Source: CAD feature listing. Evaluate the final solid. Frame: model axes, mm. A direction names the side the tool comes from. Coordinates: 2 decimals unless noted, no trailing zeros. Order: outer loops, then holes, each group sorted by start corner. A loop starts at its lowest first (then second) coordinate and runs counter-clockwise, first axis right, second up. Notation, with made-up numbers: (-39.75, 41) - (-1.75, 41) arc R30 ccw to (-1.75, 63) - close; hole circle Ø10 at (87, 77.5). An arc over 180 degrees is marked (long way). One line per question, with ' | ' between items. Start each with the question number.
(1) Section A-A (z = 0). Return the cut outline in (x, y).
(2) Section D-D (z = -46). Return the cut outline in (x, y).
(3) Access query for faces 1 (the flat face through (-251, 6, -88.9)), 2 (the flat face through (-251, 265.545, -92)), 3 (the flat face through (-251, 132.773, 92)). Directions: +Z, -Z, +X, -X, +Y, -Y. A direction counts if a zero-diameter tool reaches every point of the face in a straight line with its end or side. Return the directions, or none.
(4) Contact query for flat-ended pins moving along their axis: P1, Ø1.5, axis at x = -249, y = 214.5, coming from the -Z side; P2, Ø1.9, axis at x = -251, z = -92, coming from the -Y side; P3, Ø3, axis at x = -251.5, z = -92.5, coming from the +Y side; P4, Ø5, axis at y = 92.583, z = -37.211, coming from the -X side. Output: stop coordinate, or through.
(5) Section B-B (y = 59.5). Return the cut outline in (x, z), then the cut area to 3 significant figures.
(6) Draft query along Y for faces 4 (the flat face through (-251, 225.136, 92)), 5 (the flat face through (-251, 292.1, 92)), 6 (the flat face through (-251, 0, -86)), 7 (the flat face through (-251, 20, -95.25)). Return one class per face: +Y half, -Y half, draft (parallel to the pull), parting line (faces both ways), or undercut.
(7) Section C-C (y = 162.5). Return the cut outline in (x, z), then the cut area to 3 significant figures.
(8) Line query: line 1 along Y through (x, z) = (-248.75, 47.5); line 2 along Y through (x, z) = (-251, 17); line 3 along Y through (x, z) = (-250.25, 22.5). Output: solid intervals per line, ascending.
from build123d import *

# Parameters (mm, degrees)
SKETCH1_W           = 508
SKETCH1_H           = 190.5
BOSS_EXTRUDE1_DEPTH = 6.35
SKETCH2_W           = 508
SKETCH2_H           = 190.5
SKETCH2_W_2         = 495.3
SKETCH2_H_2         = 177.8
BOSS_EXTRUDE2_DEPTH = 298.45
SKETCH3_W           = 6.35
SKETCH3_H           = 16.933333333
SKETCH3_H_2         = 16.933333334
CUT_EXTRUDE1_DEPTH  = 12.7
SKETCH4_W           = 6.35
SKETCH4_H           = 15.875
CUT_EXTRUDE2_DEPTH  = 6.35
SKETCH6_W           = 514.801062296
SKETCH6_H           = 254.881465808
CUT_EXTRUDE5_DEPTH  = 305.8
SKETCH5_W           = 6.35
SKETCH5_H           = 16.933333333
SKETCH5_H_2         = 16.933333334
CUT_EXTRUDE6_DEPTH  = 6.35
SKETCH7_W           = 6.35
SKETCH7_H           = 12.7
CUT_EXTRUDE7_DEPTH  = 7.35
SKETCH8_R           = 26.9875
SKETCH8_R_2         = 3.175
CUT_EXTRUDE8_DEPTH  = 7.35


with BuildPart() as part:
    # Sketch1 → Boss-Extrude1 (new body)
    with BuildSketch(Plane(origin=(0, 0, 0), x_dir=(1, 0, 0), z_dir=(0, 1, 0))):
        Rectangle(SKETCH1_W, SKETCH1_H)
    extrude(amount=BOSS_EXTRUDE1_DEPTH)

    # Sketch2 → Boss-Extrude2 (add)
    with BuildSketch(Plane(origin=(0, 6.35, 0), x_dir=(1, 0, 0), z_dir=(0, 1, 0))):
        Rectangle(SKETCH2_W, SKETCH2_H)
        Rectangle(SKETCH2_W_2, SKETCH2_H_2, mode=Mode.SUBTRACT)
    extrude(amount=BOSS_EXTRUDE2_DEPTH)

    # Sketch3 → Cut-Extrude1 (cut)
    with BuildSketch(Plane.XY.offset(95.25)):
        with BuildLine():
            Line((-3.302, 283.21), (-3.302, 6.35))
            Line((-3.302, 6.35), (3.302, 6.35))
            Line((3.302, 6.35), (3.302, 292.354))
            Line((3.302, 292.354), (-16.256, 292.354))
            Line((-16.256, 292.354), (-16.256, 285.75))
            Line((-16.256, 285.75), (-5.842, 285.75))
            ThreePointArc((-5.842, 285.75), (-4.045948776, 285.006051224), (-3.302, 283.21))
        make_face()
        with Locations((12.827, 80.433333334)):
            Rectangle(SKETCH3_W, SKETCH3_H)
        with Locations((12.827, 50.8)):
            Rectangle(SKETCH3_W, SKETCH3_H_2)
        with Locations((12.827, 21.166666667)):
            Rectangle(SKETCH3_W, SKETCH3_H)
    extrude(amount=-CUT_EXTRUDE1_DEPTH, mode=Mode.SUBTRACT)

    # Sketch4 → Cut-Extrude2 (cut)
    with BuildSketch(Plane.XY.offset(-88.9)):
        with Locations((-19.431, 284.1625)):
            Rectangle(SKETCH4_W, SKETCH4_H)
        with Locations((-19.431, 255.5875)):
            Rectangle(SKETCH4_W, SKETCH4_H)
        with Locations((-19.431, 227.0125)):
            Rectangle(SKETCH4_W, SKETCH4_H)
        with Locations((-19.431, 198.4375)):
            Rectangle(SKETCH4_W, SKETCH4_H)
        with Locations((-19.431, 169.8625)):
            Rectangle(SKETCH4_W, SKETCH4_H)
        with Locations((-19.431, 141.2875)):
            Rectangle(SKETCH4_W, SKETCH4_H)
        with Locations((-19.431, 112.7125)):
            Rectangle(SKETCH4_W, SKETCH4_H)
        with Locations((-19.431, 84.1375)):
            Rectangle(SKETCH4_W, SKETCH4_H)
        with Locations((-19.431, 55.5625)):
            Rectangle(SKETCH4_W, SKETCH4_H)
        with Locations((-19.431, 26.9875)):
            Rectangle(SKETCH4_W, SKETCH4_H)
    cut_extrude2 = extrude(amount=-CUT_EXTRUDE2_DEPTH, mode=Mode.SUBTRACT)

    # Mirror1: Cut-Extrude2 across plane
    add(cut_extrude2.mirror(Plane.ZY.offset(6.477)), mode=Mode.SUBTRACT)

    # Sketch6 → Cut-Extrude5 (cut, through all)
    with BuildSketch(Plane(origin=(0, 0, 0), x_dir=(1, 0, 0), z_dir=(0, 1, 0))):
        with Locations((9.750531148, -10.000845247)):
            Rectangle(SKETCH6_W, SKETCH6_H)
    extrude(amount=CUT_EXTRUDE5_DEPTH, mode=Mode.SUBTRACT)

    # Sketch5 → Cut-Extrude6 (cut)
    with BuildSketch(Plane(origin=(0, 0, 0), x_dir=(-1, 0, 0), z_dir=(0, -1, 0))):
        with Locations((250.825, -74.083333334)):
            Rectangle(SKETCH5_W, SKETCH5_H)
        with Locations((250.825, -44.45)):
            Rectangle(SKETCH5_W, SKETCH5_H_2)
        with Locations((250.825, -14.816666667)):
            Rectangle(SKETCH5_W, SKETCH5_H)
        with Locations((250.825, 14.816666667)):
            Rectangle(SKETCH5_W, SKETCH5_H)
        with Locations((250.825, 44.45)):
            Rectangle(SKETCH5_W, SKETCH5_H_2)
        with Locations((250.825, 74.083333334)):
            Rectangle(SKETCH5_W, SKETCH5_H)
    extrude(amount=-CUT_EXTRUDE6_DEPTH, mode=Mode.SUBTRACT)

    # Sketch7 → Cut-Extrude7 (cut, through all)
    with BuildSketch(Plane.ZY.offset(254)):
        with Locations((-92.075, 32.904545455)):
            Rectangle(SKETCH7_W, SKETCH7_H)
        with Locations((-92.075, 6.35)):
            Rectangle(SKETCH7_W, SKETCH7_H)
        with Locations((-92.075, 59.459090909)):
            Rectangle(SKETCH7_W, SKETCH7_H)
        with Locations((-92.075, 86.013636364)):
            Rectangle(SKETCH7_W, SKETCH7_H)
        with Locations((-92.075, 112.568181818)):
            Rectangle(SKETCH7_W, SKETCH7_H)
        with Locations((-92.075, 139.122727273)):
            Rectangle(SKETCH7_W, SKETCH7_H)
        with Locations((-92.075, 165.677272727)):
            Rectangle(SKETCH7_W, SKETCH7_H)
        with Locations((-92.075, 192.231818182)):
            Rectangle(SKETCH7_W, SKETCH7_H)
        with Locations((-92.075, 218.786363636)):
            Rectangle(SKETCH7_W, SKETCH7_H)
        with Locations((-92.075, 245.340909091)):
            Rectangle(SKETCH7_W, SKETCH7_H)
        with Locations((-92.075, 271.895454545)):
            Rectangle(SKETCH7_W, SKETCH7_H)
        with Locations((-92.075, 298.45)):
            Rectangle(SKETCH7_W, SKETCH7_H)
        with Locations((92.075, 298.45)):
            Rectangle(SKETCH7_W, SKETCH7_H)
        with Locations((92.075, 271.895454545)):
            Rectangle(SKETCH7_W, SKETCH7_H)
        with Locations((92.075, 245.340909091)):
            Rectangle(SKETCH7_W, SKETCH7_H)
        with Locations((92.075, 218.786363636)):
            Rectangle(SKETCH7_W, SKETCH7_H)
        with Locations((92.075, 192.231818182)):
            Rectangle(SKETCH7_W, SKETCH7_H)
        with Locations((92.075, 165.677272727)):
            Rectangle(SKETCH7_W, SKETCH7_H)
        with Locations((92.075, 139.122727273)):
            Rectangle(SKETCH7_W, SKETCH7_H)
        with Locations((92.075, 112.568181818)):
            Rectangle(SKETCH7_W, SKETCH7_H)
        with Locations((92.075, 86.013636364)):
            Rectangle(SKETCH7_W, SKETCH7_H)
        with Locations((92.075, 59.459090909)):
            Rectangle(SKETCH7_W, SKETCH7_H)
        with Locations((92.075, 32.904545455)):
            Rectangle(SKETCH7_W, SKETCH7_H)
        with Locations((92.075, 6.35)):
            Rectangle(SKETCH7_W, SKETCH7_H)
    extrude(amount=-CUT_EXTRUDE7_DEPTH, mode=Mode.SUBTRACT)

    # Sketch8 → Cut-Extrude8 (cut, through all)
    with BuildSketch(Plane.ZY.offset(254)):
        with Locations((0, 55.372)):
            Circle(SKETCH8_R)
        with Locations((-37.211, 92.583)):
            Circle(SKETCH8_R_2)
        with Locations((37.211, 92.583)):
            Circle(SKETCH8_R_2)
        with Locations((37.211, 18.161)):
            Circle(SKETCH8_R_2)
        with Locations((-37.211, 18.161)):
            Circle(SKETCH8_R_2)
    extrude(amount=-CUT_EXTRUDE8_DEPTH, mode=Mode.SUBTRACT)


solid = part.part
Response values:
1) outline: (-254, 0) - (-247.65, 0) - (-247.65, 28.38) - (-254, 28.38) - close; (-254, 82.36) - (-247.65, 82.36) - (-247.65, 304.8) - (-254, 304.8) - close
2) outline: (-254, 6.35) - (-247.65, 6.35) - (-247.65, 304.8) - (-254, 304.8) - close
3) face 1: -Z, +X, -X, -Y | face 2: -Z, +X, -X | face 3: +Z, +X, -X
4) P1: stops at z = -88.9 | P2: stops at y = 12.7 | P3: stops at y = 292.1 | P4: passes through
5) outline: (-254, -88.9) - (-247.65, -88.9) - (-247.65, -26.67) - (-254, -26.67) - close; (-254, 26.67) - (-247.65, 26.67) - (-247.65, 88.9) - (-254, 88.9) - close | area: 790 mm²
6) face 4: undercut | face 5: +Y half | face 6: -Y half | face 7: draft
7) outline: (-254, -88.9) - (-247.65, -88.9) - (-247.65, 88.9) - (-254, 88.9) - close | area: 1,130 mm²
8) line 1: y = 6.35 to 304.8 | line 2: y = 6.35 to 34.41, 76.33 to 304.8 | line 3: y = 6.35 to 40.47, 70.27 to 304.8
